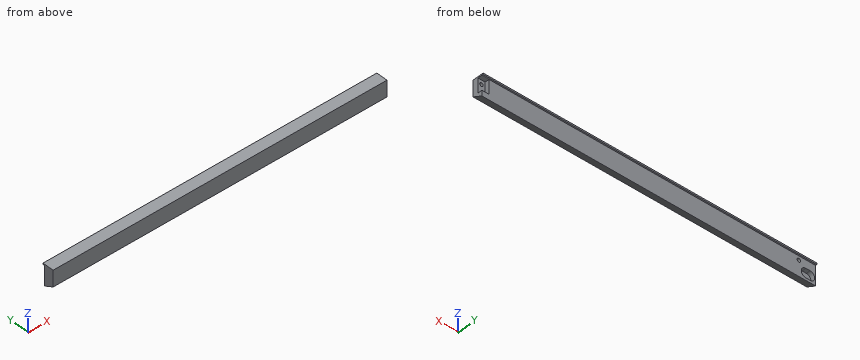
from build123d import *

# Parameters (mm, degrees)
BOX079_W               = 3
BOX079_H               = 10
BOX079_DEPTH           = 6.5
CYLINDER078_R          = 3.25
CYLINDER078_DEPTH      = 10
CYLINDER078_ROLL_ANGLE = 90
CYLINDER077_R          = 1.25
CYLINDER077_DEPTH      = 6
CYLINDER077_ROLL_ANGLE = 90
CYLINDER075_R          = 1.25
CYLINDER075_DEPTH      = 6
CYLINDER075_ROLL_ANGLE = 90
BOX078_W               = 5.1
BOX078_H               = 3.1
BOX078_DEPTH           = 10.2
CYLINDER073_R          = 3.25
CYLINDER073_DEPTH      = 10
CYLINDER073_ROLL_ANGLE = 90
BOX076_W               = 238
BOX076_H               = 8
BOX076_DEPTH           = 15
BOX074_W               = 37
BOX074_H               = 160
BOX074_DEPTH           = 120
BOX074_PITCH_ANGLE     = -15
BOX068_W               = 475
BOX068_H               = 10
BOX068_DEPTH           = 10
BOX068_ROLL_ANGLE      = -27
BOX049_W               = 475
BOX049_H               = 8
BOX049_DEPTH           = 15
BOX069_W               = 475
BOX069_H               = 8
BOX069_DEPTH           = 15


with BuildPart() as cube051:
    # Box079 → Box079 (new body)
    with BuildSketch(Plane(origin=(7, -43, 91.75), x_dir=(1, 0, 0), z_dir=(0, 0, 1))):
        with Locations((1.5, 5)):
            Rectangle(BOX079_W, BOX079_H)
    extrude(amount=BOX079_DEPTH)


with BuildPart() as fusion088:
    # Cylinder078 → Cylinder078 (new body)
    with BuildSketch(Plane.XY):
        Circle(CYLINDER078_R)
    extrude(amount=CYLINDER078_DEPTH)


with BuildPart() as fusion088_1:
    # Cylinder078 roll: moved
    add(fusion088.part.rotate(Axis((0, 0, 0), (1, 0, 0)), CYLINDER078_ROLL_ANGLE))


with BuildPart() as fusion088_2:
    # Cylinder078 placement: moved
    add(fusion088_1.part.moved(Location((10, -33, 95))))

    # Fusion088: union Cube051
    add(cube051.part)


with BuildPart() as cylinder077:
    # Cylinder077 → Cylinder077 (new body)
    with BuildSketch(Plane.XY):
        Circle(CYLINDER077_R)
    extrude(amount=CYLINDER077_DEPTH)


with BuildPart() as cylinder077_1:
    # Cylinder077 roll: moved
    add(cylinder077.part.rotate(Axis((0, 0, 0), (1, 0, 0)), CYLINDER077_ROLL_ANGLE))


with BuildPart() as cylinder077_2:
    # Cylinder077 placement: moved
    add(cylinder077_1.part.moved(Location((237.5, -40, 101))))


with BuildPart() as fusion084:
    # Cylinder075 → Cylinder075 (new body)
    with BuildSketch(Plane.XY):
        Circle(CYLINDER075_R)
    extrude(amount=CYLINDER075_DEPTH)


with BuildPart() as fusion084_1:
    # Cylinder075 roll: moved
    add(fusion084.part.rotate(Axis((0, 0, 0), (1, 0, 0)), CYLINDER075_ROLL_ANGLE))


with BuildPart() as fusion084_2:
    # Cylinder075 placement: moved
    add(fusion084_1.part.moved(Location((15, -40, 101))))

    # Fusion084: union Cylinder077
    add(cylinder077_2.part)


with BuildPart() as cube050:
    # Box078 → Box078 (new body)
    with BuildSketch(Plane(origin=(234.9, -43.1, 93.9), x_dir=(1, 0, 0), z_dir=(0, 0, 1))):
        with Locations((2.55, 1.55)):
            Rectangle(BOX078_W, BOX078_H)
    extrude(amount=BOX078_DEPTH)


with BuildPart() as cylinder073:
    # Cylinder073 → Cylinder073 (new body)
    with BuildSketch(Plane.XY):
        Circle(CYLINDER073_R)
    extrude(amount=CYLINDER073_DEPTH)


with BuildPart() as cylinder073_1:
    # Cylinder073 roll: moved
    add(cylinder073.part.rotate(Axis((0, 0, 0), (1, 0, 0)), CYLINDER073_ROLL_ANGLE))


with BuildPart() as cylinder073_2:
    # Cylinder073 placement: moved
    add(cylinder073_1.part.moved(Location((7, -33, 95))))


with BuildPart() as cube048:
    # Box076 → Box076 (new body)
    with BuildSketch(Plane(origin=(240, -47, 90), x_dir=(1, 0, 0), z_dir=(0, 0, 1))):
        with Locations((119, 4)):
            Rectangle(BOX076_W, BOX076_H)
    extrude(amount=BOX076_DEPTH)


with BuildPart() as cube046:
    # Box074 → Box074 (new body)
    with BuildSketch(Plane.XY):
        with Locations((18.5, 80)):
            Rectangle(BOX074_W, BOX074_H)
    extrude(amount=BOX074_DEPTH)


with BuildPart() as cube046_1:
    # Box074 pitch: moved
    add(cube046.part.rotate(Axis((0, 0, 0), (0, 1, 0)), BOX074_PITCH_ANGLE))


with BuildPart() as cube046_2:
    # Box074 placement: moved
    add(cube046_1.part.moved(Location((502.2, -50, -4))))


with BuildPart() as cube040:
    # Box068 → Box068 (new body)
    with BuildSketch(Plane.XY):
        with Locations((237.5, 5)):
            Rectangle(BOX068_W, BOX068_H)
    extrude(amount=BOX068_DEPTH)


with BuildPart() as cube040_1:
    # Box068 roll: moved
    add(cube040.part.rotate(Axis((0, 0, 0), (1, 0, 0)), BOX068_ROLL_ANGLE))


with BuildPart() as cube040_2:
    # Box068 placement: moved
    add(cube040_1.part.moved(Location((0, -53.1, 85.5))))


with BuildPart() as cube021:
    # Box049 → Box049 (new body)
    with BuildSketch(Plane(origin=(0, -40, 89), x_dir=(1, 0, 0), z_dir=(0, 0, 1))):
        with Locations((237.5, 4)):
            Rectangle(BOX049_W, BOX049_H)
    extrude(amount=BOX049_DEPTH)


with BuildPart() as cut095:
    # Box069 → Box069 (new body)
    with BuildSketch(Plane(origin=(0, -47, 90), x_dir=(1, 0, 0), z_dir=(0, 0, 1))):
        with Locations((237.5, 4)):
            Rectangle(BOX069_W, BOX069_H)
    extrude(amount=BOX069_DEPTH)

    # Cut066: cut Cube021
    add(cube021.part, mode=Mode.SUBTRACT)

    # Cut082: cut Cube040
    add(cube040_2.part, mode=Mode.SUBTRACT)


with BuildPart() as cut095_1:
    # Cut082 placement: moved
    add(cut095.part.moved(Location((3, 0, 0))))

    # Cut081: cut Cube046
    add(cube046_2.part, mode=Mode.SUBTRACT)

    # Cut084: cut Cube048
    add(cube048.part, mode=Mode.SUBTRACT)

    # Cut085: cut Cylinder073
    add(cylinder073_2.part, mode=Mode.SUBTRACT)

    # Cut090: cut Cube050
    add(cube050.part, mode=Mode.SUBTRACT)

    # Cut094: cut Fusion084
    add(fusion084_2.part, mode=Mode.SUBTRACT)

    # Cut095: cut Fusion088
    add(fusion088_2.part, mode=Mode.SUBTRACT)


solid = cut095_1.part
The listing builds one solid part. Answer for the finished solid, in the listing's coordinates (mm). Give positions to 0.01 mm unless a question says otherwise; leave off trailing zeros. Write each loop counter-clockwise with the first axis right and the second up, starting at its lowest first coordinate (ties: lowest second). Pieces come first, ordered by that corner, then holes.
1) Find the intervals of material crossed by L1, parallel to X at y = -43.95, z = 101; L2, parallel to Y at x = 201, z = 95.5; L3, parallel to X at y = -42.75, z = 94, in increasing order.
2) Given P1, Ø3, axis at x = 193, y = -41, coming from the -Z side; P2, Ø3.5, axis at y = -41, z = 101.5, coming from the +X side; P3, Ø4, axis at x = 237.5, z = 101, coming from the +Y side, each flat-ended and moving along its own axis, determine where each tip first touches the part or whether it passes through.
3) Section A-A (x = 193.5) is taken. Write down the section's boundary in (y, z), and give its area (3 significant figures).
Response:
1. L1: x = 3 to 13.75, 16.25 to 236.25, 238.75 to 240
1. L2: y = -47 to -40
1. L3: x = 3 to 3.91, 13.09 to 234.9
2. P1: stops at z = 90.05
2. P2: stops at x = 234.9
2. P3: stops at y = -43.1
3. outline: (-47, 93.62) - (-40, 90.05) - (-40, 104) - (-39, 104) - (-39, 105) - (-47, 105) - close
3. area: 93.2 mm2
